CAD build for the part. Positions are in the model's coordinates, mm. A direction names the side the tool comes from. Give positions to 0.01 mm unless a question says otherwise; leave off trailing zeros. Order: outer loops, then holes, each group sorted by start corner. A loop starts at its lowest first (then second) coordinate and runs counter-clockwise, first axis right, second up.
from build123d import *

# Parameters (mm, degrees)
SKETCH2_W               = 67.818
SKETCH2_H               = 27
BOSS_EXTRUDE1_DEPTH     = 5.13
SKETCH3_W               = 5.13
SKETCH3_H               = 16.6
BOSS_EXTRUDE2_DEPTH     = 5.13
CUT_EXTRUDE3_DEPTH      = 1
CUT_EXTRUDE3_DEPTH_BACK = 6.13
T_SLOT_DEPTH            = 1
T_SLOT_DEPTH_BACK       = 6.13
CUT_EXTRUDE6_DEPTH      = 1
CUT_EXTRUDE6_DEPTH_BACK = 6.13


with BuildPart() as part:
    # Sketch2 → Boss-Extrude1 (new body)
    with BuildSketch(Plane(origin=(0, 0, 0), x_dir=(0, 0, -1), z_dir=(1, 0, 0))):
        with Locations((-18.586734769, 10.276959542)):
            Rectangle(SKETCH2_W, SKETCH2_H)
    extrude(amount=BOSS_EXTRUDE1_DEPTH)

    # Sketch3 → Boss-Extrude2 (add)
    with BuildSketch(Plane(origin=(0, 23.776959542, 0), x_dir=(1, 0, 0), z_dir=(0, 1, 0))):
        with Locations((2.565, -1.986734769)):
            Rectangle(SKETCH3_W, SKETCH3_H)
        with Locations((2.565, -35.186734769)):
            Rectangle(SKETCH3_W, SKETCH3_H)
    extrude(amount=BOSS_EXTRUDE2_DEPTH)

    # Sketch6 → Cut-Extrude3 (cut, two sides)
    with BuildSketch(Plane(origin=(5.13, 0, 0), x_dir=(0, 0, -1), z_dir=(1, 0, 0))) as cut_extrude3_sk:
        Polygon((-20.085230125, 122.831802954), (-20.085230125, 23.776960132), (-20.085230125, 19.781960132), (-21.444233122, 19.781960399), (-21.444233548, 17.614960399), (-20.085233548, 17.614960132), (-20.085234769, 11.407960132), (-17.088234769, 11.407959542), (-17.088233548, 17.614959542), (-15.729233548, 17.614959275), (-15.729233122, 19.781959275), (-17.088231927, 19.781959542), (-17.088231927, 23.776959542), (-17.088231927, 122.831802365), (-17.088192956, 320.94148801), (-20.085191154, 320.9414886), align=None)
    extrude(amount=CUT_EXTRUDE3_DEPTH, mode=Mode.SUBTRACT)
    extrude(cut_extrude3_sk.sketch, amount=-CUT_EXTRUDE3_DEPTH_BACK, mode=Mode.SUBTRACT)

    # Sketch4 → t-slot (cut, two sides)
    with BuildSketch(Plane(origin=(5.13, 0, 0), x_dir=(0, 0, -1), z_dir=(1, 0, 0))) as t_slot_sk:
        Polygon((-203.979833818, 8.778464186), (-52.495735359, 8.778464186), (-48.500735359, 8.778464186), (-48.500735626, 7.419461189), (-46.333735626, 7.419460763), (-46.333735359, 8.778460763), (-40.126735359, 8.778459542), (-40.126734769, 11.775459542), (-46.333734769, 11.775460763), (-46.333734502, 13.134460763), (-48.500734502, 13.134461189), (-48.500734769, 11.775462385), (-52.495734769, 11.775462385), (-203.979833229, 11.775462385), (-506.948030149, 11.775521982), (-506.948030738, 8.778523784), align=None)
    extrude(amount=T_SLOT_DEPTH, mode=Mode.SUBTRACT)
    extrude(t_slot_sk.sketch, amount=-T_SLOT_DEPTH_BACK, mode=Mode.SUBTRACT)

    # Sketch7 → Cut-Extrude6 (cut, two sides)
    with BuildSketch(Plane(origin=(5.13, 0, 0), x_dir=(0, 0, -1), z_dir=(1, 0, 0))) as cut_extrude6_sk:
        Polygon((166.806365691, 11.775454898), (15.322265231, 11.775454898), (11.327265231, 11.775454898), (11.327265498, 13.134457895), (9.160265498, 13.134458321), (9.160265231, 11.775458321), (2.953265231, 11.775459542), (2.953264641, 8.778459542), (9.160264641, 8.778458321), (9.160264374, 7.419458321), (11.327264374, 7.419457895), (11.327264641, 8.7784567), (15.322264641, 8.7784567), (166.806365101, 8.7784567), (469.77456602, 8.778397102), (469.77456661, 11.7753953), align=None)
    extrude(amount=CUT_EXTRUDE6_DEPTH, mode=Mode.SUBTRACT)
    extrude(cut_extrude6_sk.sketch, amount=-CUT_EXTRUDE6_DEPTH_BACK, mode=Mode.SUBTRACT)


solid = part.part
1. Saw through at B-B on y = 17. Give the cut face in (x, z), plus the area to 3 significant figures.
2. Pin check, flat tips, straight feed: P1, Ø1.5, axis at y = 9, z = -1.5, coming from the -X side; P2, Ø2.5, axis at x = 4, z = -10.5, coming from the +Y side. Stop position of each tip, or through.
3. 3-axis set-ups, long thin cutter, end or side, ignore diameter. For faces 5 (the flat face through (3, 19.782, 21)), 6 (the flat face through (3, 8.778, -13)), 7 (the flat face through (3, 11.775, 43)), 8 (the flat face through (3, 23.777, -11)): which of +Z, -Z, +X, -X, +Y, -Y reach the whole face in a straight line?
4. Mould opens along Y. For faces 1 (the flat face through (3, 18, -15.322)), 2 (the flat face through (3, 11.408, 19)), 3 (the flat face through (3, 11.775, 50)), 4 (the flat face through (3, 11.775, -6)) say: released by +Y, released by -Y, zero draft, split by the parting line, or undercut.
5. Saw through at A-A on z = 44.5. Give the cut face in (x, y), plus the area to 3 significant figures.
6. Wall check: line 1 (Z direction, x = 0.4, y = 14.5); line 2 (Y direction, x = 4.75, z = 47); line 3 (Z direction, x = 0.35, y = 19.5). Give the ranges that are in metal, low to high.
Reported:
1. outline: (0, -15.32) - (5.13, -15.32) - (5.13, 17.09) - (0, 17.09) - close; (0, 20.09) - (5.13, 20.09) - (5.13, 52.5) - (0, 52.5) - close
1. area: 333 mm2
2. P1: stops at x = 0
2. P2: stops at y = 23.78
3. face 5: +X, -X
3. face 6: -Z, +X, -X
3. face 7: +Z, +X, -X
3. face 8: -Z, +X, -X, +Y
4. face 1: zero draft
4. face 2: released by +Y
4. face 3: undercut
4. face 4: undercut
5. outline: (0, -3.22) - (5.13, -3.22) - (5.13, 8.78) - (0, 8.78) - close; (0, 11.78) - (5.13, 11.78) - (5.13, 23.78) - (0, 23.78) - close
5. area: 123 mm2
6. line 1: z = -15.32 to 17.09, 20.09 to 52.5
6. line 2: y = -3.22 to 7.42, 13.13 to 23.78
6. line 3: z = -15.32 to 15.73, 21.44 to 52.5
